CAD build for the part. Positions are in the model's coordinates, mm. A direction names the side the tool comes from. Give positions to 0.01 mm unless a question says otherwise; leave off trailing zeros. Write each loop counter-clockwise with the first axis right and the second up, starting at its lowest first coordinate (ties: lowest second). Pieces come first, ordered by that corner, then holes. Notation, with made-up numbers: (-1, -27) - (54, -27) arc R26 ccw to (54, 10) - close; hole circle Ø7 at (65.5, -18). An arc over 180 degrees is marked (long way). Write item = value, one per line. Start each with the question number.
Autodesk Inventor part; units mm, degrees
ref_plane "YZ Plane" through (0, 0, 0) normal (1, 0, 0) x (0, 1, 0)
ref_plane "XZ Plane" through (0, 0, 0) normal (0, 1, 0) x (-1, 0, 0)
ref_plane "XY Plane" through (0, 0, 0) normal (0, 0, 1) x (1, 0, 0)
sketch "Sketch1" plane through (0, 0, 0) normal (0, 1, 0) x (-1, 0, 0)
  line L0 (0, 0) -> (73, 0)
  line L1 (73, 0) -> (73, -38)
  line L2 (73, -38) -> (0, -38)
  line L3 (0, -38) -> (0, 0)
  line L4 (13, -35) -> (23, -35)
  line L5 (23, -35) -> (23, -32)
  line L6 (23, -32) -> (13, -32)
  line L7 (13, -32) -> (13, -35)
  line L8 (3, -28) -> (6, -28)
  line L9 (6, -28) -> (6, -10)
  line L10 (6, -10) -> (3, -10)
  line L11 (3, -10) -> (3, -28)
  line L12 (13, -6) -> (23, -6)
  line L13 (23, -6) -> (23, -3)
  line L14 (23, -3) -> (13, -3)
  line L15 (13, -3) -> (13, -6)
  line L16 (63, -3) -> (53, -3)
  line L17 (53, -3) -> (53, -6)
  line L18 (53, -6) -> (63, -6)
  line L19 (63, -6) -> (63, -3)
  line L20 (63, -32) -> (53, -32)
  line L21 (53, -32) -> (53, -35)
  line L22 (53, -35) -> (63, -35)
  line L23 (63, -35) -> (63, -32)
  point P0 (3, -19)
  point P1 (0, -19)
  dimension "d0" = 73
  dimension "d1" = 38
  dimension "d3" = 3
  dimension "d4" = 3
  dimension "d5" = 3
  dimension "d6" = 10
  dimension "d7" = 10
  dimension "d8" = 18
  dimension "d9" = 32
  dimension "d10" = 3
  dimension "d11" = 3
  dimension "d12" = 3
  dimension "d13" = 10
  dimension "d14" = 13
extrude "Extrusion1" add sketch "Sketch1" along normal blind 3
fillet "Fillet1" radius 3 2 edges at (0, 1.5, 0) (0, 1.5, -38)
sketch "Sketch2" plane through (0, 0, 0) normal (0, -1, 0) x (1, 0, 0)
  line L0 (-3, -10) -> (-3, -28)
  line L1 (-3, -28) -> (-6, -28)
  line L2 (-6, -28) -> (-6, -10)
  line L3 (-6, -10) -> (-3, -10)
  line L4 (-63, -35) -> (-63, -32)
  line L5 (-63, -32) -> (-53, -32)
  line L6 (-53, -32) -> (-53, -35)
  line L7 (-53, -35) -> (-63, -35)
  line L8 (-63, -6) -> (-63, -3)
  line L9 (-63, -3) -> (-53, -3)
  line L10 (-53, -3) -> (-53, -6)
  line L11 (-53, -6) -> (-63, -6)
  line L12 (-13, -3) -> (-13, -6)
  line L13 (-13, -6) -> (-23, -6)
  line L14 (-23, -6) -> (-23, -3)
  line L15 (-23, -3) -> (-13, -3)
  line L16 (-13, -32) -> (-13, -35)
  line L17 (-13, -35) -> (-23, -35)
  line L18 (-23, -35) -> (-23, -32)
  line L19 (-23, -32) -> (-13, -32)
  arc A0 (-3, -38) -> (0, -35) centre (-3, -35) ccw
  line L20 (0, -35) -> (0, -3)
  arc A1 (0, -3) -> (-3, 0) centre (-3, -3) ccw
  line L21 (-3, 0) -> (-73, 0)
  line L22 (-73, 0) -> (-73, -38)
  line L23 (-73, -38) -> (-3, -38)
  line L24 (-9.5, -15) -> (-21.5, -15) construction
  line L25 (-11.5, -17) -> (-19.5, -17)
  line L26 (-19.5, -13) -> (-11.5, -13)
  arc A2 (-11.5, -17) -> (-11.5, -13) centre (-11.5, -15) ccw
  arc A3 (-19.5, -13) -> (-19.5, -17) centre (-19.5, -15) ccw
  line L27 (-73, 0) -> (-73, -38)
  point P0 (0, 0)
  point P1 (-73, -19)
  point P2 (-15.5, -15)
  point P3 (-73, -19)
  dimension "d21" = 2
  dimension "d22" = 8
  dimension "d23" = 11.5
  dimension "d26" = 15
extrude "Extrusion2" cut sketch "Sketch2" against normal blind 3 contours L25 A3 L26 A2
sketch "Sketch3" plane through (0, 3, 0) normal (0, 1, 0) x (1, 0, 0)
  arc A0 (-11.5, 13) -> (-11.5, 17) centre (-11.5, 15) ccw
  line L0 (-11.5, 13) -> (-19.5, 13)
  arc A1 (-19.5, 17) -> (-19.5, 13) centre (-19.5, 15) ccw
  line L1 (-19.5, 17) -> (-11.5, 17)
  arc A2 (0, 35) -> (-3, 38) centre (-3, 35) ccw
  line L2 (-3, 38) -> (-73, 38)
  line L3 (-73, 38) -> (-73, 0)
  line L4 (-73, 0) -> (-3, 0)
  arc A3 (-3, 0) -> (0, 3) centre (-3, 3) ccw
  line L5 (0, 3) -> (0, 35)
  line L6 (-3, 28) -> (-3, 10)
  line L7 (-3, 10) -> (-6, 10)
  line L8 (-6, 10) -> (-6, 28)
  line L9 (-6, 28) -> (-3, 28)
  line L10 (-63, 32) -> (-63, 35)
  line L11 (-63, 35) -> (-53, 35)
  line L12 (-53, 35) -> (-53, 32)
  line L13 (-53, 32) -> (-63, 32)
  line L14 (-63, 3) -> (-63, 6)
  line L15 (-63, 6) -> (-53, 6)
  line L16 (-53, 6) -> (-53, 3)
  line L17 (-53, 3) -> (-63, 3)
  line L18 (-13, 6) -> (-13, 3)
  line L19 (-13, 3) -> (-23, 3)
  line L20 (-23, 3) -> (-23, 6)
  line L21 (-23, 6) -> (-13, 6)
  line L22 (-13, 35) -> (-13, 32)
  line L23 (-13, 32) -> (-23, 32)
  line L24 (-23, 32) -> (-23, 35)
  line L25 (-23, 35) -> (-13, 35)
  point P0 (0, 0)
equation "\"d5\" = d4"
equation "\"d10\" = d11"
properties part number "motor mount top" material "Polycarbonate, Clear"
1. Tool access for faces 1 (the cylindrical face through (-0.9, 1.52, -0.86)), 2 (the flat face through (-18, 1, -35)): list every direction of +Z, -Z, +X, -X, +Y, -Y with a clear straight run to the whole face (end or side of a thin tool).
2. Wall check: line 1 along X through (y, z) = (1.5, -5); line 2 along Z through (x, y) = (-12, 1.55); line 3 along X through (y, z) = (0.2, -15). Give the ranges that are in metal, low to high.
3. Cut at D-D (z = -25.5). Give the cut face in (x, y).
4. Cut at C-C (y = 0.5). Count the separate pieces of the cut face and the enclosed holes in it, then the cut area to 3 significant figures.
5. Mould opens along X. For faces 3 (the flat face through (-18, 1, -3)), 4 (the cylindrical face through (-0.86, 1.52, -37.1)), 5 (the flat face through (-38, 1, 0)) say: +X half, -X half, draft (parallel to the pull), parting line (faces both ways), or undercut.
6. Cut at A-A (x = -58). Give the cut face in (y, z).
7. Cut at B-B (x = -18.5). Give the cut face in (y, z).
Output:
q1.face_1 = +Z, +X, +Y, -Y
q1.face_2 = +Y, -Y
q2.line_1 = -73 to -63, -53 to -23, -13 to 0
q2.line_2 = -38 to -17, -13 to 0
q2.line_3 = -73 to -21.5, -9.5 to -6, -3 to 0
q3.outline = (-73, 0) - (-6, 0) - (-6, 3) - (-73, 3) - close; (-3, 0) - (0, 0) - (0, 3) - (-3, 3) - close
q4.separate_pieces = 1
q4.enclosed_holes = 6
q4.area = 2,550 mm2
q5.face_3 = undercut
q5.face_4 = +X half
q5.face_5 = draft
q6.outline = (0, -38) - (3, -38) - (3, -35) - (0, -35) - close; (0, -32) - (3, -32) - (3, -6) - (0, -6) - close; (0, -3) - (3, -3) - (3, 0) - (0, 0) - close
q7.outline = (0, -38) - (3, -38) - (3, -35) - (0, -35) - close; (0, -32) - (3, -32) - (3, -17) - (0, -17) - close; (0, -13) - (3, -13) - (3, -6) - (0, -6) - close; (0, -3) - (3, -3) - (3, 0) - (0, 0) - close
